Could you check a few things on this model? Use its own coordinates, in mm. Give positions to 0.01 mm unless a question says otherwise; leave off trailing zeros. Write each loop counter-clockwise with the first axis right and the second up, starting at its lowest first coordinate (ties: lowest second). Pieces come first, ordered by that corner, then holes. Notation, with made-up numbers: (-27.5, 72.5) - (-16.5, 72.5) arc R29 cw to (-16.5, 92.5) - close; hole circle Ø1 at (-27.5, -16). An arc over 180 degrees is marked (long way). Answer as CSV lines item,"result". Start each with the question number.
Q1. If I drill on line 1 along Y through (x, z) = (25.5, -0.25); line 2 along Y through (x, z) = (46.5, -1); line 3 along Z through (x, y) = (46, 5.5), over which ranges is the centre line in solid material (lowest first)?
Q2. Will these pins go through, and if not, where does the flat tip stop? pin 1 Ø6 at (x, y) = (34, 4.5) entering from -Z; pin 2 Ø1.5 at (x, y) = (23.5, -2) entering from +Z; pin 3 Ø2 at (y, z) = (-5, -1) entering from -X; pin 4 Ø2 at (x, z) = (39.5, 2.5) entering from -Y.
Q3. Imagine slicing it at A-A on x = 29. List the corners of the cut face in (y, z) for me.
Autodesk Inventor part; units mm, degrees
ref_plane "YZ Plane" through (0, 0, 0) normal (1, 0, 0) x (0, 1, 0)
ref_plane "XZ Plane" through (0, 0, 0) normal (0, 1, 0) x (-1, 0, 0)
ref_plane "XY Plane" through (0, 0, 0) normal (0, 0, 1) x (1, 0, 0)
sketch "Sketch1" plane through (0, 0, 0) normal (1, 0, 0) x (0, 1, 0)
  circle A0 centre (0, 0) radius 7
  dimension "d0" = 14
extrude "Extrusion1" add sketch "Sketch1" along normal blind 64
chamfer "Chamfer1" distance 2 angle 45 1 edges at (64, -7, 0) measured on face at (64, -0.8274, 0.9129)
chamfer "Chamfer2" distance 2 angle 45 1 edges at (0, -7, 0) measured on face at (0, -0.8274, 0.9129)
properties part number "Stub" material "Steel, Carbon"
Conclusion:
1,line 1,"-7 to 7"
1,line 2,"-6.93 to 6.93"
1,line 3,"-4.33 to 4.33"
2,pin 1,"z = -6.84"
2,pin 2,"z = 6.89"
2,pin 3,"x = 0"
2,pin 4,"y = -6.84"
3,outline,"circle Ø14 at (0, 0)"
